Job drawing, mm, ordinate dimensions from the low corner. One solid piece. A direction names the side the tool comes from. Give positions to 0.01 mm unless a question says otherwise; leave off trailing zeros. Write each loop counter-clockwise with the first axis right and the second up, starting at its lowest first coordinate (ties: lowest second). Pieces come first, ordered by that corner, then holes. Notation, with made-up numbers: M 32.5,70.5 L 67.5,70.5 A21 ccw 67.5,78.5 Z; hole C -8,81 d11. An arc over 180 degrees is marked long. Use a Markdown table: item, result.
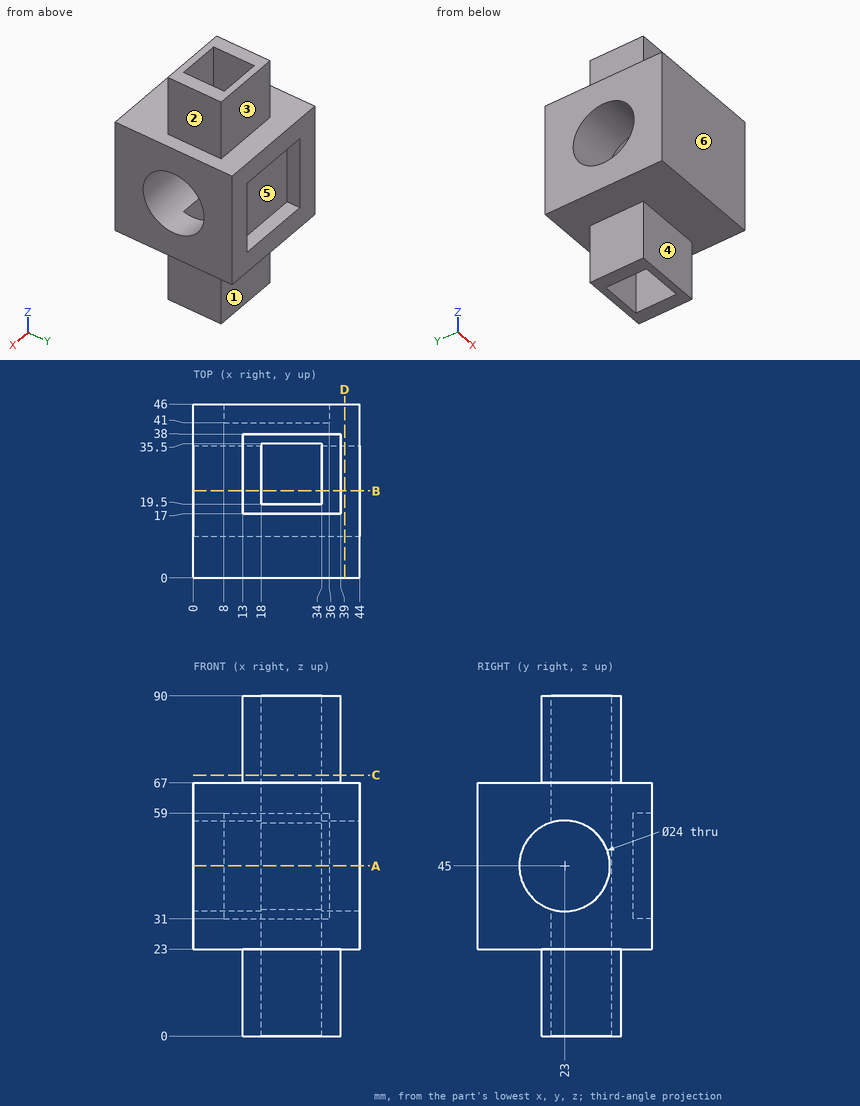
1. Drill centre lines: L1, parallel to Y at x = 27.5, z = 20; L2, parallel to Y at x = 20, z = 45; L3, parallel to X at y = 30.5, z = 63. Where is each one in solid material? Low to high.
Findings below:
| item | result |
|---|---|
| L1 | 17 to 19.5, 35.5 to 38 |
| L2 | 0 to 11, 35.5 to 41 |
| L3 | 0 to 18, 34 to 44 |
2. Cut at D-D, the plane x = 40. Give the cut face in (y, z).
Findings below:
| item | result |
|---|---|
| outline | M 0,23 L 46,23 L 46,67 L 0,67 Z; hole C 23,45 d24 |
3. Two-plate mould, pull along Z, no slides. Class the marked faces 5 and 6: released by +Z, released by -Z, zero draft, split by the parting line, or undercut.
Findings below:
| item | result |
|---|---|
| face 5 | undercut |
| face 6 | zero draft |
4. Cut at B-B, the plane y = 23. Give the cut face in (x, z).
Findings below:
| item | result |
|---|---|
| outline | M 0,23 L 13,23 L 13,0 L 18,0 L 18,33 L 0,33 Z; M 0,57 L 18,57 L 18,90 L 13,90 L 13,67 L 0,67 Z; M 34,0 L 39,0 L 39,23 L 44,23 L 44,33 L 34,33 Z; M 34,57 L 44,57 L 44,67 L 39,67 L 39,90 L 34,90 Z |
5. Tool access for the marked faces 1, 2, 3 and 4: list every direction of +Z, -Z, +X, -X, +Y, -Y with a clear straight run to the whole face (end or side of a thin tool).
Findings below:
| item | result |
|---|---|
| face 1 | -Z, +X, -X, +Y |
| face 2 | +Z, +X, +Y, -Y |
| face 3 | +Z, +X, -X, +Y |
| face 4 | -Z, +X, -X, -Y |
6. Cut at A-A, the plane z = 45. Give the cut face in (x, y).
Findings below:
| item | result |
|---|---|
| outline | M 0,0 L 44,0 L 44,11 L 0,11 Z; M 0,35 L 18,35 L 18,35.5 L 34,35.5 L 34,35 L 44,35 L 44,46 L 36,46 L 36,41 L 8,41 L 8,46 L 0,46 Z |
7. Drop flat-ended pins along their axis: P1, Ø6.5, axis at y = 27, z = 14.5, coming from the -X side; P2, Ø7, axis at x = 29, z = 82, coming from the -Y side; P3, Ø13, axis at x = 29, z = 80.5, coming from the +Y side; P4, Ø10, axis at x = 8, z = 42.5, coming from the -Y side. Give the stop position or say it passes through.
Findings below:
| item | result |
|---|---|
| P1 | x = 13 |
| P2 | y = 17 |
| P3 | y = 38 |
| P4 | y = 0 |
8. Cut at C-C, the plane z = 69. Give the cut face in (x, y).
Findings below:
| item | result |
|---|---|
| outline | M 13,17 L 39,17 L 39,38 L 13,38 Z; hole M 18,19.5 L 34,19.5 L 34,35.5 L 18,35.5 Z |
